Autodesk Inventor part; units mm, degrees
ref_plane "Plano de trabajo1" through (0, 97.4, 0) normal (0, 1, 0) x (-1, 0, 0)
ref_plane "YZ Plane" through (0, 0, 0) normal (1, 0, 0) x (0, 1, 0)
ref_plane "XY Plane" through (0, 0, 0) normal (0, 0, 1) x (1, 0, 0)
sketch "Boceto1" plane through (0, 0, 0) normal (0, 1, 0) x (-1, 0, 0)
  circle A0 centre (0, 0) radius 9.25
  dimension "d0" = 18.5
ref_plane "Plano de trabajo1" through (0, 97.4, 0) normal (0, 1, 0) x (-1, 0, 0)
sketch "Boceto2" plane through (0, 97.4, 0) normal (0, 1, 0) x (-1, 0, 0)
  circle A0 centre (0, 0) radius 8.5
  dimension "d2" = 17
loft "Solevación1" add profiles "Boceto2", "Boceto1"
sketch "Boceto3" plane through (0, 97.4, 0) normal (0, 1, 0) x (1, 0, 0)
  circle A0 centre (0, 0) radius 8.5
  circle A1 centre (0, 0) radius 4.35
  dimension "d7" = 8.7
extrude "Extrusión1" add sketch "Boceto3" along normal blind 17.1 contours A1
fillet "Empalme1" radius 2 1 edges at (8.5, 97.4, 0)
sketch "Boceto4" plane through (0, 114.5, 0) normal (0, 1, 0) x (1, 0, 0)
  line L0 (-2.95, -1.92) -> (2.95, -1.92)
  line L1 (2.95, -1.92) -> (2.95, 1.92)
  line L2 (2.95, 1.92) -> (-2.95, 1.92)
  line L3 (-2.95, 1.92) -> (-2.95, -1.92)
  line L4 (-2.95, -1.92) -> (2.95, 1.92) construction
  line L5 (2.95, -1.92) -> (-2.95, 1.92) construction
  point P0 (0, 0)
  dimension "d11" = 5.9
  dimension "d12" = 3.84
extrude "Extrusión2" add sketch "Boceto4" along normal blind 4.5
sketch "Boceto5" plane through (-2.95, 114.5, 1.92) normal (0, 0, 1) x (1, 0, 0)
  line L0 (5.9, 4.5) -> (0, 4.5)
  line L1 (0, 4.5) -> (0, 7)
  line L2 (5.9, 0) -> (5.9, 4.5)
  line L3 (0, 7) -> (5.9, 4.5)
  line L4 (5.9, 4.5) -> (0, 4.5)
  point P0 (2.95, -114.5)
  dimension "d15" = 2.5
extrude "Extrusión3" add sketch "Boceto5" against normal up to surface (3.84 mm away)
sketch "Boceto6" plane through (0, 0, 0) normal (0, -1, 0) x (1, 0, 0)
  circle A0 centre (0, 0) radius 7
  line L0 (0, -7) -> (0, -4.3)
  line L1 (0, -4.3) -> (0.65, -4.3012)
  circle A1 centre (0, 0) radius 4.35
  line L2 (0.65, -4.3012) -> (0.6452, -6.9702)
  line L3 (0, -4.3) -> (-0.65, -4.3)
  line L4 (0, -4.3) -> (0.65, -4.3) construction
  line L5 (-0.65, -4.3) -> (-0.65, -6.9698)
  line L6 (-2.5818, -3.501) -> (-4.4724, -5.3849)
  line L7 (-3.0406, -3.0406) -> (-2.5809, -3.5002) construction
  line L8 (-3.0406, -3.0406) -> (-3.5002, -2.5809)
  line L9 (-3.5002, -2.5809) -> (-5.388, -4.4687)
  line L10 (-3.0406, -3.0406) -> (-2.5818, -3.501)
  line L11 (-4.3012, -0.65) -> (-6.9702, -0.6452)
  line L12 (-4.3, 0) -> (-4.3, -0.65) construction
  line L13 (-4.3, 0) -> (-4.3, 0.65)
  line L14 (-4.3, 0.65) -> (-6.9698, 0.65)
  line L15 (-4.3, 0) -> (-4.3012, -0.65)
  line L16 (-3.501, 2.5818) -> (-5.3849, 4.4724)
  line L17 (-3.0406, 3.0406) -> (-3.5002, 2.5809) construction
  line L18 (-3.0406, 3.0406) -> (-2.5809, 3.5002)
  line L19 (-2.5809, 3.5002) -> (-4.4687, 5.388)
  line L20 (-3.0406, 3.0406) -> (-3.501, 2.5818)
  line L21 (-0.65, 4.3012) -> (-0.6452, 6.9702)
  line L22 (0, 4.3) -> (-0.65, 4.3) construction
  line L23 (0, 4.3) -> (0.65, 4.3)
  line L24 (0.65, 4.3) -> (0.65, 6.9698)
  line L25 (0, 4.3) -> (-0.65, 4.3012)
  line L26 (2.5818, 3.501) -> (4.4724, 5.3849)
  line L27 (3.0406, 3.0406) -> (2.5809, 3.5002) construction
  line L28 (3.0406, 3.0406) -> (3.5002, 2.5809)
  line L29 (3.5002, 2.5809) -> (5.388, 4.4687)
  line L30 (3.0406, 3.0406) -> (2.5818, 3.501)
  line L31 (4.3012, 0.65) -> (6.9702, 0.6452)
  line L32 (4.3, 0) -> (4.3, 0.65) construction
  line L33 (4.3, 0) -> (4.3, -0.65)
  line L34 (4.3, -0.65) -> (6.9698, -0.65)
  line L35 (4.3, 0) -> (4.3012, 0.65)
  line L36 (3.501, -2.5818) -> (5.3849, -4.4724)
  line L37 (3.0406, -3.0406) -> (3.5002, -2.5809) construction
  line L38 (3.0406, -3.0406) -> (2.5809, -3.5002)
  line L39 (2.5809, -3.5002) -> (4.4687, -5.388)
  line L40 (3.0406, -3.0406) -> (3.501, -2.5818)
  dimension "d18" = 14
  dimension "d19" = 2.7
  dimension "d20" = 0.65
  dimension "d21" = 90
  dimension "d22" = 0.65
  dimension "d23" = 180
  dimension "d24" = 90
  dimension "d27" = 360
extrude "Extrusión4" cut sketch "Boceto6" against normal blind 10 contours L31 A1 L29 A0 | A0 L36 A1 L34 | L35 L33 A1 L40 L38 L1 L3 L10 L8 L15 L13 L20 L18 L25 L23 L30 L28 | L26 A1 L24 A0 | A0 L2 A1 L39 | L21 A1 L19 A0 | A0 L6 A1 L5 | L16 A1 L14 A0 | A0 L11 A1 L9
properties part number "Marcador" material "Madera (arce)"
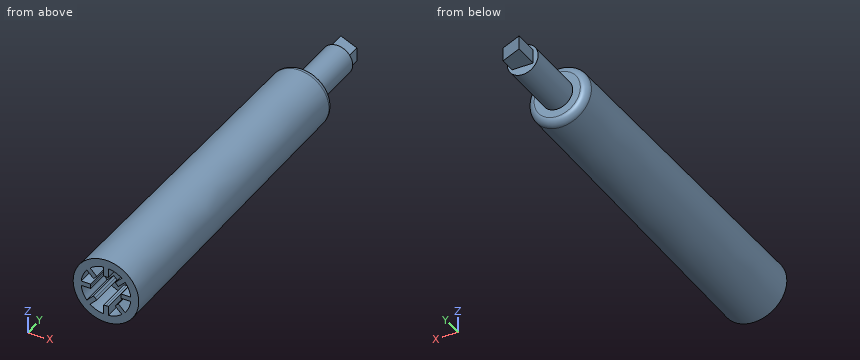
Geometry: final body of the model. Coordinates: model frame, mm. Give positions to 0.01 mm unless a question says otherwise; leave off trailing zeros. Write each loop counter-clockwise with the first axis right and the second up, starting at its lowest first coordinate (ties: lowest second). Pieces come first, ordered by that corner, then holes.
1. Line query: probe 1 along Z at (x, y) = (2.25, 6); probe 2 along Y at (x, z) = (-5.25, -0.25); probe 3 along Y at (x, z) = (-5, 2). Output: solid intervals per line, ascending.
2. Section query A-A, the plane y = 89.5. Return loops of the section in (x, z).
3. Section query B-B, the plane y = 35.5. Return loops of the section in (x, z).
4. Pin query (flat end, axial travel): P1, Ø1.9, axis at y = 116.5, z = -1, coming from the +X side; P2, Ø1, axis at y = 52.5, z = -2, coming from the +X side; P3, Ø6, axis at y = 92, z = -1.5, coming from the -X side. Return the tip coordinate at first contact, or that it passes through.
Computed:
1. probe 1: z = -8.92 to -6.63, 6.63 to 8.92
1. probe 2: y = 0 to 97.4
1. probe 3: y = 10 to 97.4
2. outline: circle Ø17.12 at (0, 0)
3. outline: circle Ø17.95 at (0, 0)
4. P1: stops at x = 2.95
4. P2: stops at x = 8.72
4. P3: stops at x = -8.56
